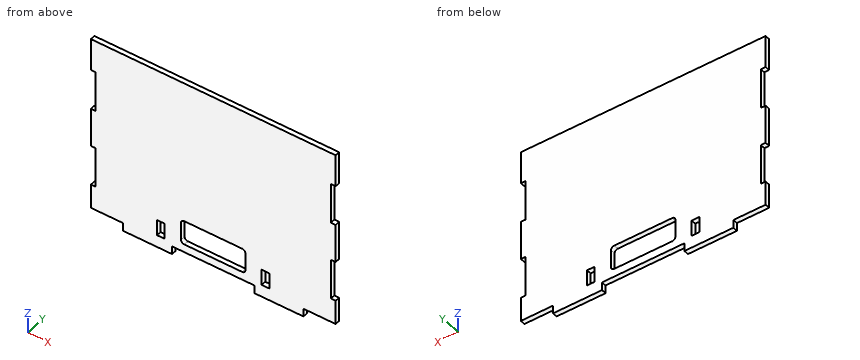
from build123d import *

# Parameters (mm, degrees)
BOSS_EXTRUDE1_DEPTH = 3
SKETCH2_W           = 4.8
SKETCH2_H           = 9.8
CUT_EXTRUDE1_DEPTH  = 96.047356618


with BuildPart() as part:
    # Sketch1 → Boss-Extrude1 (new body)
    with BuildSketch(Plane(origin=(0, 0, 0), x_dir=(1, 0, 0), z_dir=(0, 1, 0))):
        Polygon((0, 52), (0, -57), (-76, -57), (-76, -37), (-73, -37), (-73, -12), (-76, -12), (-76, 12), (-73, 12), (-73, 37), (-76, 37), (-76, 52), (-56, 52), (-56, 57), (-25.6, 57), (-25.6, 52), align=None)
    boss_extrude1 = extrude(amount=BOSS_EXTRUDE1_DEPTH)

    # Mirror1: Boss-Extrude1 across plane
    add(boss_extrude1.mirror(Plane(origin=(0, 3, -52), x_dir=(0, 0, 1), z_dir=(-1, 0, 0))))

    # Sketch2 → Cut-Extrude1 (cut, through all)
    with BuildSketch(Plane(origin=(0, 3, 0), x_dir=(1, 0, 0), z_dir=(0, 1, 0))):
        with Locations((-32.5, 44.5)):
            Rectangle(SKETCH2_W, SKETCH2_H)
        with Locations((32.5, 44.5)):
            Rectangle(SKETCH2_W, SKETCH2_H)
        with BuildLine():
            Line((-18, 47), (18, 47))
            ThreePointArc((18, 47), (19.414213562, 46.414213562), (20, 45))
            Line((20, 45), (20, 34))
            ThreePointArc((20, 34), (19.414213562, 32.585786438), (18, 32))
            Line((18, 32), (-18, 32))
            ThreePointArc((-18, 32), (-19.414213562, 32.585786438), (-20, 34))
            Line((-20, 34), (-20, 45))
            ThreePointArc((-20, 45), (-19.414213562, 46.414213562), (-18, 47))
        make_face()
    extrude(amount=-CUT_EXTRUDE1_DEPTH, mode=Mode.SUBTRACT)


solid = part.part
Here's how the part is built. I have some questions about the finished solid (model axes, mm). Give positions to 0.01 mm unless a question says otherwise; leave off trailing zeros. Loops run counter-clockwise (first coordinate to the right, second up) from the corner with the lowest first, then second, coordinate; pieces in that order, holes last. Notation, with made-up numbers: (-12.5, 75.25) -> (14.5, 75.25) arc R28 ccw to (14.5, 93.25) -> close; hole circle Ø8 at (-25, 37). An arc over 180 degrees is marked (long way). Answer as a JSON object with one key per item and string values. Group by question number.
Item 1: Imagine slicing it at D-D on x = -64.5. Write out the boundary of the cut face in (y, z).
Item 2: Imagine slicing it at B-B on y = 1.95. Give the number of separate pieces and of enclosed holes in the cut face, then the cut area to 3 significant figures.
Item 3: Imagine slicing it at A-A on x = -2. Write out the boundary of the cut face in (y, z).
Item 4: I need wall thicknesses on L1, parallel to Z at x = -13.5, y = 1.95; L2, parallel to X at y = 1.9, z = -39; L3, parallel to X at y = 0.6, z = -28.5. Which ranges of each line are inside material? Lowest first, please.
Item 5: Will these pins go through, and if not, where does the flat tip stop? pin 1 (0.9 mm diameter, centred on y = 2, z = 26.5, fed in from +X); pin 2 (0.9 mm diameter, centred on x = 1, y = 2, fed in from -Z); pin 3 (4 mm diameter, centred on x = -44, z = -18, fed in from -Y).
Item 6: Imagine slicing it at C-C on z = -28. Write out the boundary of the cut face in (x, y).
Answer list:
{
 "1": {"outline": "(0, -52) -> (3, -52) -> (3, 57) -> (0, 57) -> close"},
 "2": {"separate pieces": "1", "enclosed holes": "3", "area": "15,900 mm2"},
 "3": {"outline": "(0, -52) -> (3, -52) -> (3, -47) -> (0, -47) -> close; (0, -32) -> (3, -32) -> (3, 57) -> (0, 57) -> close"},
 "4": {"L1": "z = -52 to -47, -32 to 57", "L2": "x = -76 to -20, 20 to 76", "L3": "x = -73 to 73"},
 "5": {"pin 1": "stops at x = 73", "pin 2": "stops at z = -52", "pin 3": "stops at y = 0"},
 "6": {"outline": "(-73, 0) -> (73, 0) -> (73, 3) -> (-73, 3) -> close"}
}
